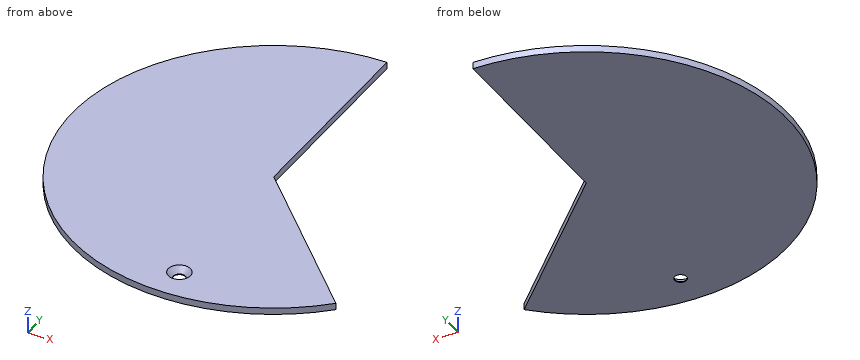
```python
from build123d import *

# Parameters (mm, degrees)
BOSS_EXTRUDE1_DEPTH = 2.54


with BuildPart() as part:
    # Sketch1 → Boss-Extrude1 (new body)
    with BuildSketch(Plane.XY):
        with BuildLine():
            Line((0, 0), (53.881536726, -53.881536726))
            ThreePointArc((53.881536726, -53.881536726), (-70.399620377, -29.160477546), (0, 76.2))
            Line((0, 76.2), (0, 0))
        make_face()
    extrude(amount=BOSS_EXTRUDE1_DEPTH)

    # Sketch3 → CSK for #8 Flat Head Machine Screw1 (revolve, cut)
    with BuildSketch(Plane(origin=(0, -63.5, 2.54), x_dir=(0, -1, 0), z_dir=(1, 0, 0))):
        Polygon((0, 0), (0, 2.54), (2.2479, 2.54), (2.2479, 2.26450021), (4.2164, 0), align=None)
    revolve(axis=Axis((0, -63.5, 8.89), (0, 0, -1)), mode=Mode.SUBTRACT)


solid = part.part
```
Could you check a few things on this model? Use its own coordinates, in mm. Give positions to 0.01 mm unless a question says otherwise; leave off trailing zeros. Loops run counter-clockwise (first coordinate to the right, second up) from the corner with the lowest first, then second, coordinate; pieces in that order, holes last. Notation, with made-up numbers: (10, -26.75) - (65, -26.75) arc R6 cw to (65, -18.75) - close; hole circle Ø1 at (68, 52). An arc over 180 degrees is marked (long way). Use one line per item in the form item = value.
1. I need wall thicknesses on probe 1 along X at (y, z) = (-63.5, 0.2); probe 2 along X at (y, z) = (29.5, 2.4); probe 3 along Y at (x, z) = (-21, 2.35). Which ranges of each line are inside material? Lowest first, please.
Response values:
probe_1 = -42.12 to -2.25, 2.25 to 42.12
probe_2 = -70.26 to 0
probe_3 = -73.25 to 73.25
2. I want a section at A-A (y = -63.5). Please give me the cut outline in (x, z).
Response values:
outline = (-42.12, 0) - (-2.25, 0) - (-2.25, 0.28) - (-4.22, 2.54) - (-42.12, 2.54) - close; (2.25, 0) - (42.12, 0) - (42.12, 2.54) - (4.22, 2.54) - (2.25, 0.28) - close
3. I want a section at C-C (y = 28). Please give me the cut outline in (x, z), and give its area (3 significant figures).
Response values:
outline = (-70.87, 0) - (0, 0) - (0, 2.54) - (-70.87, 2.54) - close
area = 180 mm²
4. I'm going to push a flat-ended pin straight in: pin 1 Ø1.5 at (y, z) = (59, 2) entering from +X. Where does the tip first touch, or does it pass through?
Response values:
pin_1 = 0
5. I want a section at B-B (x = -36.5). Please give me the cut outline in (y, z), and give its area (3 significant figures).
Response values:
outline = (-66.89, 0) - (66.89, 0) - (66.89, 2.54) - (-66.89, 2.54) - close
area = 340 mm²
